from build123d import *

# Parameters (mm, degrees)
ESQUISSE1_W             = 130
ESQUISSE1_H             = 65
ESQUISSE1_R             = 1.3
BOSS_EXTRU_1_DEPTH      = 5
ESQUISSE2_W             = 130
ESQUISSE2_H             = 12.5
ESQUISSE2_H_2           = 22
ENL_V_MAT_EXTRU_1_DEPTH = 0.5
D_GAGEMENT_M3_D         = 3.4
D_GAGEMENT_M3_DEPTH     = 6.978536948
D_GAGEMENT_M3_TIP       = 1.021463052
D_GAGEMENT_M32_D        = 3.4
D_GAGEMENT_M32_DEPTH    = 6.978536948
D_GAGEMENT_M32_TIP      = 1.021463052


with BuildPart() as part:
    # Esquisse1 → Boss.-Extru.1 (new body)
    with BuildSketch(Plane.XY):
        with Locations((65, 32.5)):
            Rectangle(ESQUISSE1_W, ESQUISSE1_H)
        with Locations((113, 5)):
            Circle(ESQUISSE1_R, mode=Mode.SUBTRACT)
        with Locations((89, 5)):
            Circle(ESQUISSE1_R, mode=Mode.SUBTRACT)
        with Locations((65, 5)):
            Circle(ESQUISSE1_R, mode=Mode.SUBTRACT)
        with Locations((41, 5)):
            Circle(ESQUISSE1_R, mode=Mode.SUBTRACT)
        with Locations((17, 5)):
            Circle(ESQUISSE1_R, mode=Mode.SUBTRACT)
        with Locations((113, 60)):
            Circle(ESQUISSE1_R, mode=Mode.SUBTRACT)
        with Locations((89, 60)):
            Circle(ESQUISSE1_R, mode=Mode.SUBTRACT)
        with Locations((65, 60)):
            Circle(ESQUISSE1_R, mode=Mode.SUBTRACT)
        with Locations((41, 60)):
            Circle(ESQUISSE1_R, mode=Mode.SUBTRACT)
        with Locations((17, 60)):
            Circle(ESQUISSE1_R, mode=Mode.SUBTRACT)
    extrude(amount=BOSS_EXTRU_1_DEPTH)

    # Esquisse2 → Enlèv. mat.-Extru.1 (cut)
    with BuildSketch(Plane(origin=(0, 0, 0), x_dir=(-1, 0, 0), z_dir=(0, 0, -1))):
        with Locations((-65, 58.75)):
            Rectangle(ESQUISSE2_W, ESQUISSE2_H)
        with Locations((-65, 6.25)):
            Rectangle(ESQUISSE2_W, ESQUISSE2_H)
        with Locations((-65, 32.5)):
            Rectangle(ESQUISSE2_W, ESQUISSE2_H_2)
    extrude(amount=-ENL_V_MAT_EXTRU_1_DEPTH, mode=Mode.SUBTRACT)

    # Dégagement M3
    with Locations(Plane.XY.offset(5)):
        with Locations((17, 60), (41, 60), (65, 60), (89, 60), (113, 60), (113, 5), (89, 5), (65, 5), (41, 5), (17, 5)):
            Hole(D_GAGEMENT_M3_D / 2, depth=D_GAGEMENT_M3_DEPTH)
            with Locations((0, 0, -(D_GAGEMENT_M3_DEPTH + D_GAGEMENT_M3_TIP / 2))):  # 118° drill point
                Cone(0, D_GAGEMENT_M3_D / 2, D_GAGEMENT_M3_TIP, mode=Mode.SUBTRACT)

    # Dégagement M32
    with Locations(Plane(origin=(0, 0, 0.5), x_dir=(-1, 0, 0), z_dir=(0, 0, -1))):
        with Locations((-125, 55), (-101, 55), (-77, 55), (-53, 55), (-29, 55), (-5, 55), (-40, 32.5), (-90, 32.5), (-125, 10), (-101, 10), (-77, 10), (-53, 10), (-29, 10), (-5, 10)):
            Hole(D_GAGEMENT_M32_D / 2, depth=D_GAGEMENT_M32_DEPTH)
            with Locations((0, 0, -(D_GAGEMENT_M32_DEPTH + D_GAGEMENT_M32_TIP / 2))):  # 118° drill point
                Cone(0, D_GAGEMENT_M32_D / 2, D_GAGEMENT_M32_TIP, mode=Mode.SUBTRACT)


solid = part.part
Input: part model. Units: mm. Frame: model coordinates. A direction names the side the tool comes from. Coordinates: 2 decimals unless noted, no trailing zeros. Loops run counter-clockwise (first coordinate to the right, second up) from the corner with the lowest first, then second, coordinate; pieces in that order, holes last.
(1) Section C-C on z = 3.55. Count the separate pieces of the cut face and the enclosed holes in it, then the cut area to 3 significant figures.
(2) Section B-B on y = 55. Return the cut outline in (x, z), then the cut area to 3 significant figures.
(3) First-contact query: pin 1 Ø3 at (x, y) = (89, 5) entering from -Z; pin 2 Ø4 at (x, y) = (29, 10) entering from -Z; pin 3 Ø5.5 at (x, y) = (65, 5) entering from +Z. Flat tips, straight axial feed; report the tip coordinate or a pass-through.
(4) Pull-direction query (X, two-part tool) for faces 1 (the face through (130, 32, 2)), 2 (the face through (99.3, 10.07, 2.78)), 3 (the face through (64, 65, 3)); classes: released by +X, released by -X, zero draft, split by the parting line, or undercut.
(5) Material intervals for probe 1 along Y at (x, z) = (29, 3.7); probe 2 along Y at (x, z) = (17, 1.5); probe 3 along Z at (x, y) = (73, 36), sorted ascending.
(6) Set-up query: faces 4 (the face through (66, 33, 0.5)), 5 (the face through (66, 8, 0.5)), 6 (the face through (64, 17, 0)). Return all of +Z, -Z, +X, -X, +Y, -Y with unobstructed straight access to the full face (end or side cutting, diameter ignored); none if empty.
(7) Section A-A on x = 65. Return the cut outline in (y, z).
(8) Section D-D on y = 41. Return the cut outline in (x, z).
Data:
1. separate pieces: 1
1. enclosed holes: 24
1. area: 8,230 mm2
2. outline: (0, 0.5) - (3.3, 0.5) - (3.3, 5) - (0, 5) - close; (6.7, 0.5) - (27.3, 0.5) - (27.3, 5) - (6.7, 5) - close; (30.7, 0.5) - (51.3, 0.5) - (51.3, 5) - (30.7, 5) - close; (54.7, 0.5) - (75.3, 0.5) - (75.3, 5) - (54.7, 5) - close; (78.7, 0.5) - (99.3, 0.5) - (99.3, 5) - (78.7, 5) - close; (102.7, 0.5) - (123.3, 0.5) - (123.3, 5) - (102.7, 5) - close; (126.7, 0.5) - (130, 0.5) - (130, 5) - (126.7, 5) - close
2. area: 493 mm2
3. pin 1: passes through
3. pin 2: stops at z = 0.5
3. pin 3: stops at z = 5
4. face 1: released by +X
4. face 2: undercut
4. face 3: zero draft
5. probe 1: y = 0 to 8.3, 11.7 to 53.3, 56.7 to 65
5. probe 2: y = 0 to 3.3, 6.7 to 58.3, 61.7 to 65
5. probe 3: z = 0.5 to 5
6. face 4: -Z, +X, -X
6. face 5: -Z, +X, -X, -Y
6. face 6: -Z, +X, -X, +Y, -Y
7. outline: (0, 0.5) - (3.3, 0.5) - (3.3, 5) - (0, 5) - close; (6.7, 0.5) - (12.5, 0.5) - (12.5, 0) - (21.5, 0) - (21.5, 0.5) - (43.5, 0.5) - (43.5, 0) - (52.5, 0) - (52.5, 0.5) - (58.3, 0.5) - (58.3, 5) - (6.7, 5) - close; (61.7, 0.5) - (65, 0.5) - (65, 5) - (61.7, 5) - close
8. outline: (0, 0.5) - (130, 0.5) - (130, 5) - (0, 5) - close
